CAD build for the part. Positions are in the model's coordinates, mm. Face numbers are marked on the shaded views. A direction names the side the tool comes from. Give positions to 0.01 mm unless a question says otherwise; leave off trailing zeros. Loops run counter-clockwise (first coordinate to the right, second up) from the corner with the lowest first, then second, coordinate; pieces in that order, holes last. Notation, with made-up numbers: M 29.25,-29 L 72.25,-29 A26 cw 72.25,4 Z; hole C -12.75,-30.5 d10. An arc over 180 degrees is marked long. Answer as CSV lines item,"result".
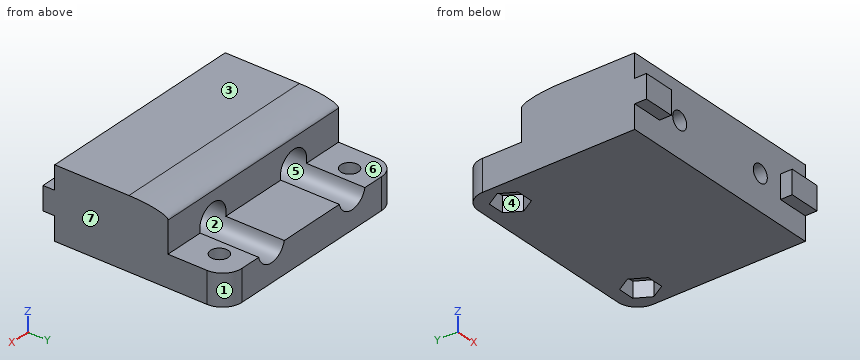
from build123d import *

# Parameters (mm, degrees)
SKETCH_1_W          = 55
SKETCH_1_H          = 18
EXTRUDE_1_DEPTH     = 44
SKETCH_2_R          = 2.25
CUT_EXTRUDE_1_DEPTH = 40
SKETCH_3_R          = 2.25
CUT_EXTRUDE_2_DEPTH = 50
SKETCH_4_R          = 4.25
CUT_EXTRUDE_3_DEPTH = 22
CUT_EXTRUDE_START   = -4
SKETCH_5_R          = 2.25
CUT_EXTRUDE_4_DEPTH = 4
FILLET_1_R          = 5
SKETCH_6_W          = 8
SKETCH_6_H          = 6
EXTRUDE_2_DEPTH     = 3
SKETCH_7_W          = 71.435921238
SKETCH_7_H          = 28.786378212
CUT_EXTRUDE_5_DEPTH = 10
FILLET_2_SIZE       = 10
FILLET_2_SIZE_2     = 2


with BuildPart() as part:
    # Эскиз1 → Бобышка-Вытянуть1 (new body)
    with BuildSketch(Plane(origin=(0, 0, 0), x_dir=(1, 0, 0), z_dir=(0, 1, 0))):
        with Locations((27.5, 9)):
            Rectangle(SKETCH_1_W, SKETCH_1_H)
    extrude(amount=EXTRUDE_1_DEPTH)

    # Эскиз2 → Вырез-Вытянуть1 (cut)
    with BuildSketch(Plane.XY):
        with Locations((48.5, 37)):
            Circle(SKETCH_2_R)
        with Locations((6.5, 37)):
            Circle(SKETCH_2_R)
    extrude(amount=-CUT_EXTRUDE_1_DEPTH, mode=Mode.SUBTRACT)

    # Эскиз3 → Вырез-Вытянуть2 (cut)
    with BuildSketch(Plane(origin=(0, 44, 0), x_dir=(1, 0, 0), z_dir=(0, 1, 0))):
        with Locations(Location((40.5, 9, 0), (0, 0, 270))):
            Circle(SKETCH_3_R)
        with Locations(Location((14.5, 9, 0), (0, 0, 90))):
            Circle(SKETCH_3_R)
    extrude(amount=-CUT_EXTRUDE_2_DEPTH, mode=Mode.SUBTRACT)

    # Эскиз4 → Вырез-Вытянуть3 (cut)
    with BuildSketch(Plane(origin=(0, 44, 0), x_dir=(1, 0, 0), z_dir=(0, 1, 0))):
        with Locations(Location((40.5, 9, 0), (0, 0, 270))):
            Circle(SKETCH_4_R)
        with Locations(Location((14.5, 9, 0), (0, 0, 270))):
            Circle(SKETCH_4_R)
    extrude(amount=-CUT_EXTRUDE_3_DEPTH, mode=Mode.SUBTRACT)

    # Эскиз5 → Вырез-Вытянуть4 (cut)
    # profile 1 of 2: a face of its own
    with BuildSketch(Plane(origin=(0, 0, -18), x_dir=(-1, 0, 0), z_dir=(0, 0, -1)).offset(CUT_EXTRUDE_START)):
        Polygon((-52.772391992, 37), (-50.636195996, 33.3), (-46.363804004, 33.3), (-44.227608008, 37), (-46.363804004, 40.7), (-50.636195996, 40.7), align=None)
        with Locations((-48.5, 37)):
            Circle(SKETCH_5_R, mode=Mode.SUBTRACT)
    # profile 2 of 2: a face of its own
    with BuildSketch(Plane(origin=(0, 0, -18), x_dir=(-1, 0, 0), z_dir=(0, 0, -1)).offset(CUT_EXTRUDE_START)):
        Polygon((-10.772391992, 37), (-8.636195996, 33.3), (-4.363804004, 33.3), (-2.227608008, 37), (-4.363804004, 40.7), (-8.636195996, 40.7), align=None)
        with Locations(Location((-6.5, 37, 0), (0, 0, 180))):
            Circle(SKETCH_5_R, mode=Mode.SUBTRACT)
    extrude(amount=CUT_EXTRUDE_4_DEPTH, mode=Mode.SUBTRACT)

    # Скругление1
    fillet_1_edges = [part.edges().sort_by_distance(p)[0] for p in [
        (55, 44, -9),
        (0, 44, -9),
    ]]
    fillet(fillet_1_edges, radius=FILLET_1_R)

    # Эскиз6 → Бобышка-Вытянуть2 (add)
    with BuildSketch(Plane.XZ):
        with Locations((51, -9)):
            Rectangle(SKETCH_6_W, SKETCH_6_H)
        with Locations((4, -9)):
            Rectangle(SKETCH_6_W, SKETCH_6_H)
    extrude(amount=EXTRUDE_2_DEPTH)

    # Эскиз7 → Вырез-Вытянуть5 (cut)
    with BuildSketch(Plane.XY):
        with Locations((35.717960619, 43.393189106)):
            Rectangle(SKETCH_7_W, SKETCH_7_H)
    extrude(amount=-CUT_EXTRUDE_5_DEPTH, mode=Mode.SUBTRACT)

    # Скругление2
    # an asymmetric fillet: 10, 2 mm, written as the material it takes off along each edge
    with BuildSketch(Plane(origin=(-25, 29, 0), x_dir=(0, -1, 0), z_dir=(1, 0, 0))) as fillet_2_piece_1:
        with BuildLine():
            Bezier((FILLET_2_SIZE, 0), (0, 0), (0, FILLET_2_SIZE_2), weights=[1, 0.707106781, 1])
            Line((0, FILLET_2_SIZE_2), (0, 0))
            Line((0, 0), (FILLET_2_SIZE, 0))
        make_face()
    extrude(amount=105, mode=Mode.SUBTRACT)


solid = part.part
1) Mould opens along Z. For the marked faces 1, 2 and 3 say: +Z half, -Z half, draft (parallel to the pull), parting line (faces both ways), or undercut.
Answer below:
face 1,"draft"
face 2,"undercut"
face 3,"+Z half"
2) Band-saw the part on A-A on y = 36. Give the cut face in (x, z).
Answer below:
outline,"M 0,-18 L 2.8,-18 L 2.8,-14 L 4.48,-14 L 4.48,-10 L 0,-10 Z; M 8.52,-14 L 10.2,-14 L 10.2,-18 L 44.8,-18 L 44.8,-14 L 46.48,-14 L 46.48,-10 L 44.63,-10 A4.25 cw 36.37,-10 L 18.63,-10 A4.25 cw 10.37,-10 L 8.52,-10 Z; M 50.52,-14 L 52.2,-14 L 52.2,-18 L 55,-18 L 55,-10 L 50.52,-10 Z"
3) Which spindle directions (+Z, -Z, +X, -X, +Y, -Y) get a long thin tool onto all of the face, cutting with end or side? Do the marked faces 4, 5, 6 and 7. Say none if no direction does.
Answer below:
face 4,"-Z"
face 5,"+Y"
face 6,"+Z, +X, -X, +Y"
face 7,"+Z, -Z, +X, +Y, -Y"
4) Band-saw the part on B-B on y = 5.5. Give the cut face in (x, z).
Answer below:
outline,"M 0,-18 L 55,-18 L 55,0 L 0,0 Z; hole C 14.5,-9 d4.5; hole C 40.5,-9 d4.5"
5) Band-saw the part on C-C on z = -3. Give the cut face in (x, y), and give its area (4 significant figures).
Answer below:
outline,"M 0,0 L 55,0 L 55,29 L 0,29 Z"
area,"1,595 mm^2"
6) Flat gauge pins, fed straight in: pin 1 (7 mm diameter, centred on x = 14.5, z = -9, fed in from -Y); pin 2 (5 mm diameter, centred on x = 40.5, z = -9, fed in from +Y); pin 3 (7.5 mm diameter, centred on x = 28, y = 34.5, fed in from +Z). Where does each tip first touch, or does it go through?
Answer below:
pin 1,"stops at y = 0"
pin 2,"stops at y = 22"
pin 3,"stops at z = -10"
7) Drill centre lines: line 1 (Z direction, x = 14.5, y = 9.5); line 2 (Y direction, x = 6.5, z = -12.4); line 3 (X direction, y = 37, z = -12.35). Where is each one in solid material? Low to high. Write a range as from..to.
Answer below:
line 1,"z = -18..-11.25, -6.75..0"
line 2,"y = 0..34.75, 39.25..44"
line 3,"x = 0..4.25, 8.75..11.88, 17.12..37.88, 43.12..46.25, 50.75..55"
8) Band-saw the part on D-D on y = 25. Give the number of separate pieces and of enclosed holes in the cut face, and give its area (3 significant figures).
Answer below:
separate pieces,"1"
enclosed holes,"2"
area,"855 mm^2"
